```python
from build123d import *

# Parameters (mm, degrees)
SKETCH1_R   = 6
SKETCH1_R_2 = 4.8
COIL1_DEPTH = 1.2
SKETCH2_R   = 6
SKETCH2_R_2 = 4.8
COIL2_DEPTH = 1.2
SKETCH3_R   = 6
SKETCH3_R_2 = 4.8
COIL3_DEPTH = 1.2
SKETCH4_R   = 6
SKETCH4_R_2 = 4.8
COIL4_DEPTH = 1.2
SKETCH5_R   = 6
SKETCH5_R_2 = 4.8
COIL5_DEPTH = 1.2
SKETCH6_R   = 6
SKETCH6_R_2 = 4.8
COIL6_DEPTH = 1.2
SKETCH7_W   = 1
SKETCH7_H   = 1
LINK1_DEPTH = 1.8
SKETCH8_W   = 1
SKETCH8_H   = 1
LINK2_DEPTH = 1.8
SKETCH9_W   = 1
SKETCH9_H   = 1
LINK3_DEPTH = 1.8
SKETCH10_W  = 1
SKETCH10_H  = 1
LINK4_DEPTH = 1.8
SKETCH11_W  = 1
SKETCH11_H  = 1
LINK5_DEPTH = 1.8


with BuildPart() as part:
    # Sketch1 → Coil1 (new body)
    with BuildSketch(Plane.XY):
        Circle(SKETCH1_R)
        Circle(SKETCH1_R_2, mode=Mode.SUBTRACT)
    extrude(amount=COIL1_DEPTH)



with BuildPart() as body_2:
    # Sketch2 → Coil2 (new body)
    with BuildSketch(Plane.XY.offset(3)):
        Circle(SKETCH2_R)
        Circle(SKETCH2_R_2, mode=Mode.SUBTRACT)
    extrude(amount=COIL2_DEPTH)


with BuildPart() as body_3:
    # Sketch3 → Coil3 (new body)
    with BuildSketch(Plane.XY.offset(6)):
        Circle(SKETCH3_R)
        Circle(SKETCH3_R_2, mode=Mode.SUBTRACT)
    extrude(amount=COIL3_DEPTH)


with BuildPart() as body_4:
    # Sketch4 → Coil4 (new body)
    with BuildSketch(Plane.XY.offset(9)):
        Circle(SKETCH4_R)
        Circle(SKETCH4_R_2, mode=Mode.SUBTRACT)
    extrude(amount=COIL4_DEPTH)


with BuildPart() as body_5:
    # Sketch5 → Coil5 (new body)
    with BuildSketch(Plane.XY.offset(12)):
        Circle(SKETCH5_R)
        Circle(SKETCH5_R_2, mode=Mode.SUBTRACT)
    extrude(amount=COIL5_DEPTH)


with BuildPart() as body_6:
    # Sketch6 → Coil6 (new body)
    with BuildSketch(Plane.XY.offset(15)):
        Circle(SKETCH6_R)
        Circle(SKETCH6_R_2, mode=Mode.SUBTRACT)
    extrude(amount=COIL6_DEPTH)


with BuildPart() as part_1:
    add(part.part)

    add(body_2.part)  # Link1 merges body 2
    # Sketch7 → Link1 (add)
    with BuildSketch(Plane.XY.offset(1.2)):
        with Locations((5.4, 0)):
            Rectangle(SKETCH7_W, SKETCH7_H)
    extrude(amount=LINK1_DEPTH)


    add(body_3.part)  # Link2 merges body 3
    # Sketch8 → Link2 (add)
    with BuildSketch(Plane.XY.offset(4.2)):
        with Locations((-5.4, 0)):
            Rectangle(SKETCH8_W, SKETCH8_H)
    extrude(amount=LINK2_DEPTH)


    add(body_4.part)  # Link3 merges body 4
    # Sketch9 → Link3 (add)
    with BuildSketch(Plane.XY.offset(7.2)):
        with Locations((5.4, 0)):
            Rectangle(SKETCH9_W, SKETCH9_H)
    extrude(amount=LINK3_DEPTH)


    add(body_5.part)  # Link4 merges body 5
    # Sketch10 → Link4 (add)
    with BuildSketch(Plane.XY.offset(10.2)):
        with Locations((-5.4, 0)):
            Rectangle(SKETCH10_W, SKETCH10_H)
    extrude(amount=LINK4_DEPTH)


    add(body_6.part)  # Link5 merges body 6
    # Sketch11 → Link5 (add)
    with BuildSketch(Plane.XY.offset(13.2)):
        with Locations((5.4, 0)):
            Rectangle(SKETCH11_W, SKETCH11_H)
    extrude(amount=LINK5_DEPTH)


solid = part_1.part
```
For this review, take the finished solid that the model builds, in its own axes (mm). A direction names the side the tool comes from. Coordinates: 2 decimals unless noted, no trailing zeros. Write each loop counter-clockwise with the first axis right and the second up, starting at its lowest first coordinate (ties: lowest second). Pieces come first, ordered by that corner, then holes. Notation, with made-up numbers: (-15.75, 77.25) - (-1.75, 77.25) arc R17 cw to (-1.75, 85.25) - close; hole circle Ø3 at (42.25, 70). An arc over 180 degrees is marked (long way). Answer in a Markdown table with one row per item. Add a question column.
Q1. For probe 1 along Z at (x, y) = (2.75, 5); probe 2 along Y at (x, z) = (0, 0.9); probe 3 along Y at (x, z) = (5, 8.25), list the stretches that pass through material, from the lowest coordinate up.
Q2. Draft analysis for pull direction X (two halves, no side actions). For faces 6 (the flat face through (5.4, 0.5, 2.1)), 7 (the flat face through (-4.9, 0, 5)), 8 (the cylindrical face through (2.58, 4.05, 15.59)), state which applies: +X half, -X half, draft (parallel to the pull), parting line (faces both ways), or undercut.
Q3. Tool access review of faces 1 (the cylindrical face through (-6, 0, 13)), 2 (the flat face through (-5.4, -0.5, 11.1)), 3 (the flat face through (-5.4, 0.5, 5.1)), 4 (the flat face through (-5.9, 0, 11)), 5 (the flat face through (5.9, 0, 2)): name each direction out of +Z, -Z, +X, -X, +Y, -Y from which nothing blocks a thin tool from reaching the whole face with its end or side.
Q4. We need section A-A, the plane x = 0. Count the separate pieces of the cut face and the enclosed holes in it, and give its area (3 significant figures).
Q5. For P1, Ø3.5, axis at x = -1.5, y = 1.5, coming from the +Z side; P2, Ø6, axis at x = -4.5, z = 5, coming from the +Y side; P3, Ø0.8, axis at y = 0, z = 11, coming from the -X side; P4, Ø1, axis at y = -3.5, z = 3, coming from the +X side, all flat-tipped, find the tip position at first contact; note any pin that passes through.
Q6. We need section C-C, the plane z = 2. State the section outline as (x, y) points, and give its area (3 significant figures).
Q7. We need section D-D, the plane z = 6.25. State the section outline as (x, y) points.
Answer list:
| question | item | result |
|---|---|---|
| 1 | probe 1 | z = 0 to 1.2, 3 to 4.2, 6 to 7.2, 9 to 10.2, 12 to 13.2, 15 to 16.2 |
| 1 | probe 2 | y = -6 to -4.8, 4.8 to 6 |
| 1 | probe 3 | y = -0.5 to 0.5 |
| 2 | face 6 | draft |
| 2 | face 7 | +X half |
| 2 | face 8 | undercut |
| 3 | face 1 | +Z, -Z |
| 3 | face 2 | +X, -X, -Y |
| 3 | face 3 | +X, -X, +Y |
| 3 | face 4 | -X, +Y, -Y |
| 3 | face 5 | +X, +Y, -Y |
| 4 | separate pieces | 12 |
| 4 | enclosed holes | 0 |
| 4 | area | 17.3 mm2 |
| 5 | P1 | passes through |
| 5 | P2 | stops at y = 5.78 |
| 5 | P3 | stops at x = -5.9 |
| 5 | P4 | stops at x = 5.2 |
| 6 | outline | (4.9, -0.5) - (5.9, -0.5) - (5.9, 0.5) - (4.9, 0.5) - close |
| 6 | area | 1.00 mm2 |
| 7 | outline | circle Ø12 at (0, 0); hole circle Ø9.6 at (0, 0) |
